Work out the finished part from the listing and answer in its coordinate system (mm). Face numbers are marked on the shaded views. A direction names the side the tool comes from. Round coordinates to 2 decimals unless told otherwise and drop trailing zeros. Loops run counter-clockwise (first coordinate to the right, second up) from the corner with the lowest first, then second, coordinate; pieces in that order, holes last. Notation, with made-up numbers: (-18.5, 20) -> (6.5, 20) arc R18 ccw to (6.5, 47) -> close; hole circle Ø11 at (-3, -31). An arc over 180 degrees is marked (long way). Use CSV: the item, a comma, the result in double quotes. Start each with the question number.
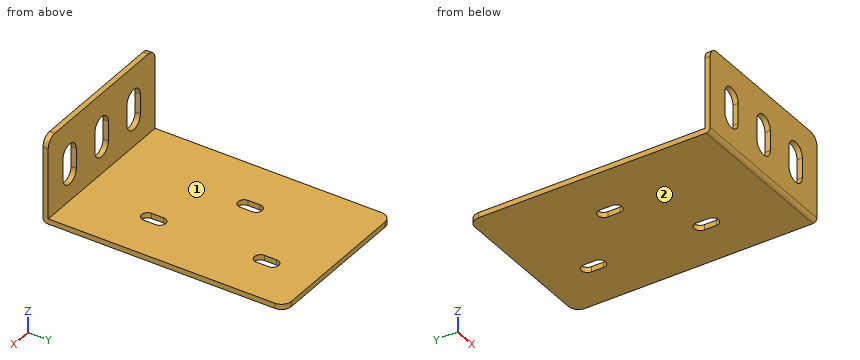
from build123d import *

# Parameters (mm, degrees)
F0_W     = 50.8
F0_H     = 76.2
F1_DEPTH = 1.651
F2_W     = 50.8
F2_H     = 1.651
F3_DEPTH = 25.4
F4_R     = 1.27
F5_R     = 3.175
F6_W     = 1.905
F6_H     = 3.81
F7_DEPTH = 25.4
F9_DEPTH = 25.4


# Not quite as in the source:
# - a feature names something its author has since deleted; it is built from what else it names


with BuildPart() as f1:
    # F0 (on Top) → F1 (new body)
    with BuildSketch(Plane.XY):
        with Locations((0, -3.81)):
            Rectangle(F0_W, F0_H)
    extrude(amount=F1_DEPTH)

    # F2 (on face) → F3 (join)
    with BuildSketch(Plane.XY.offset(1.651)):
        with Locations((0, -41.0845)):
            Rectangle(F2_W, F2_H)
    extrude(amount=F3_DEPTH)

    # F4
    f4_edges = [f1.edges().sort_by_distance(p)[0] for p in [
        (0, -41.91, 0),
    ]]
    fillet(f4_edges, radius=F4_R)

    # F5
    f5_edges = [f1.edges().sort_by_distance(p)[0] for p in [
        (25.4, 34.29, 0.8255),
        (-25.4, 34.29, 0.8255),
        (25.4, -41.0845, 27.051),
        (-25.4, -41.0845, 27.051),
    ]]
    fillet(f5_edges, radius=F5_R)

    # F6 (on face) → F7 (cut)
    with BuildSketch(Plane.XY.offset(1.651)):
        with BuildLine():
            Line((-6.985, -1.27), (-6.985, 2.54))
            ThreePointArc((-6.985, 2.54), (-8.89, 4.445), (-10.795, 2.54))
            Line((-10.795, 2.54), (-8.89, 2.54))
            Line((-8.89, 2.54), (-8.89, -1.27))
            Line((-8.89, -1.27), (-10.795, -1.27))
            ThreePointArc((-10.795, -1.27), (-8.89, -3.175), (-6.985, -1.27))
        make_face()
        with Locations((-9.8425, 0.635)):
            Rectangle(F6_W, F6_H)
        with BuildLine():
            ThreePointArc((8.255, 16.51), (10.16, 14.605), (12.065, 16.51))
            Line((12.065, 16.51), (12.065, 20.32))
            ThreePointArc((12.065, 20.32), (10.16, 22.225), (8.255, 20.32))
            Line((8.255, 20.32), (8.255, 16.51))
        make_face()
        with BuildLine():
            ThreePointArc((12.065, -15.24), (10.16, -13.335), (8.255, -15.24))
            Line((8.255, -15.24), (8.255, -19.05))
            ThreePointArc((8.255, -19.05), (10.16, -20.955), (12.065, -19.05))
            Line((12.065, -19.05), (12.065, -15.24))
        make_face()
    extrude(amount=-F7_DEPTH, mode=Mode.SUBTRACT)

    # F8 (on face) → F9 (cut)
    with BuildSketch(Plane.XZ.offset(41.91)):
        with BuildLine():
            ThreePointArc((-12.065, 16.51), (-15.24, 19.685), (-18.415, 16.51))
            Line((-18.415, 16.51), (-18.415, 10.16))
            ThreePointArc((-18.415, 10.16), (-15.24, 6.985), (-12.065, 10.16))
            Line((-12.065, 10.16), (-12.065, 16.51))
        make_face()
        with BuildLine():
            Line((3.175, 10.16), (3.175, 16.51))
            ThreePointArc((3.175, 16.51), (0, 19.685), (-3.175, 16.51))
            Line((-3.175, 16.51), (-3.175, 10.16))
            ThreePointArc((-3.175, 10.16), (0, 6.985), (3.175, 10.16))
        make_face()
        with BuildLine():
            Line((18.415, 10.16), (18.415, 16.51))
            ThreePointArc((18.415, 16.51), (15.24, 19.685), (12.065, 16.51))
            Line((12.065, 16.51), (12.065, 10.16))
            ThreePointArc((12.065, 10.16), (15.24, 6.985), (18.415, 10.16))
        make_face()
    extrude(amount=-F9_DEPTH, mode=Mode.SUBTRACT)


solid = f1.part
Q1. Section A-A, the plane x = 0 is taken. Write down the section's boundary in (y, z) (3 decimals), and give its area (3 significant figures).
Q2. Straight lines are drawn through the part: line 1 (Z direction, x = -8, y = -15); line 2 (Y direction, x = -10.5, z = 9.25). For each, find the intervals that lie inside material, in ascending order. Write a range as from..to.
Q3. Each of these flat-tipped pins is pushed along its axis until it touches: pin 1 (12.5 mm diameter, centred on x = 5, z = 10.5, fed in from +Y); pin 2 (15 mm diameter, centred on x = 11, y = -11, fed in from +Z); pin 3 (8 mm diameter, centred on y = 8, z = 8.5, fed in from +X). Where does it stop, or does it pass through?
Q4. Section C-C, the plane x = -8.89 is taken. Write down the section's boundary in (y, z) (3 decimals), and give its area (3 significant figures).
Q5. Which of the six approach directions +Z, -Z, +X, -X, +Y, -Y give full straight-line access (tool end or side, diameter ignored) to the marked faces 1 and 2?
Q6. Section B-B, the plane x = 10.16 is taken. Write down the section's boundary in (y, z) (3 decimals).
Q7. Section D-D, the plane y = 13 is taken. Write down the section's boundary in (x, z), and give its area (3 significant figures).
Report:
1,outline,"(-41.91, 1.27) arc R1.27 ccw to (-40.64, 0) -> (34.29, 0) -> (34.29, 1.651) -> (-40.259, 1.651) -> (-40.259, 6.985) -> (-41.91, 6.985) -> close; (-41.91, 19.685) -> (-40.259, 19.685) -> (-40.259, 27.051) -> (-41.91, 27.051) -> close"
1,area,"146 mm²"
2,line 1,"z = 0..1.65"
2,line 2,"y = -41.91..-40.26"
3,pin 1,"stops at y = -40.26"
3,pin 2,"stops at z = 1.65"
3,pin 3,"passes through"
4,outline,"(-41.91, 1.27) arc R1.27 ccw to (-40.64, 0) -> (-3.175, 0) -> (-3.175, 1.651) -> (-40.259, 1.651) -> (-40.259, 27.051) -> (-41.91, 27.051) -> close; (4.445, 0) -> (34.29, 0) -> (34.29, 1.651) -> (4.445, 1.651) -> close"
4,area,"155 mm²"
5,face 1,"+Z, +X, -X, +Y"
5,face 2,"-Z, +X, -X, +Y, -Y"
6,outline,"(-41.91, 1.27) arc R1.27 ccw to (-40.64, 0) -> (-20.955, 0) -> (-20.955, 1.651) -> (-40.259, 1.651) -> (-40.259, 27.051) -> (-41.91, 27.051) -> close; (-13.335, 0) -> (14.605, 0) -> (14.605, 1.651) -> (-13.335, 1.651) -> close; (22.225, 0) -> (34.29, 0) -> (34.29, 1.651) -> (22.225, 1.651) -> close"
7,outline,"(-25.4, 0) -> (25.4, 0) -> (25.4, 1.65) -> (-25.4, 1.65) -> close"
7,area,"83.9 mm²"
